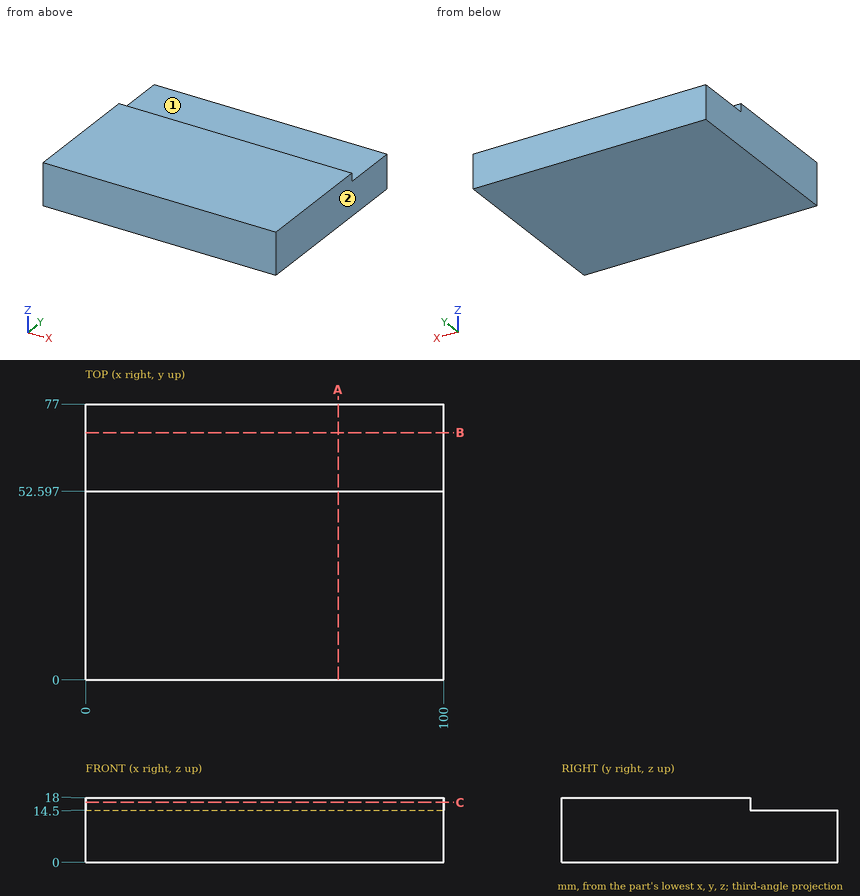
Study the drawing (mm; zero at the part's minimum x, y, z) and answer. A direction names the side the tool comes from. Give positions to 0.01 mm unless a question says otherwise; leave off trailing zeros. Order: outer loops, then holes, each group sorted by start corner. A loop starts at its lowest first (then second) coordinate and runs counter-clockwise, first axis right, second up. Notation, with made-up numbers: (49.25, 14) - (90.25, 14) arc R22 cw to (90.25, 40) - close; hole circle Ø9 at (-28.75, -37.75). An arc over 180 degrees is marked (long way). Use one line per item in the form item = value. Start each with the question number.
(1) A cutting plane is placed at A-A, the plane x = 70.5. Write down the section's boundary in (y, z).
(2) Consider line 1 (Z direction, x = 24, y = 66.5); line 2 (Y direction, x = 17, z = 17). Determine where each line is inside the solid, lowest interval first. Write a range as from..to.
(3) A cutting plane is placed at C-C, the plane z = 16.75. Write down the section's boundary in (x, y), then the cut area to 3 significant figures.
(4) A cutting plane is placed at B-B, the plane y = 69. Write down the section's boundary in (x, z).
(5) Flat-ended cylindrical pins translate along their axes: pin 1 Ø4 at (y, z) = (11.5, 4.5) entering from -X; pin 2 Ø1 at (x, z) = (49, 16) entering from +Y; pin 3 Ø7.5 at (x, y) = (29.5, 60.5) entering from +Z. Find the tip coordinate at first contact, or state that the pin passes through.
(6) For the marked faces 1 and 2, determine the directions among +Z, -Z, +X, -X, +Y, -Y from which every point of the face is accessible in a straight line to the end or side of a thin tool.
Ans:
q1.outline = (0, 0) - (77, 0) - (77, 14.5) - (52.6, 14.5) - (52.6, 18) - (0, 18) - close
q2.line_1 = 0..14.5
q2.line_2 = 0..52.6
q3.outline = (0, 0) - (100, 0) - (100, 52.6) - (0, 52.6) - close
q3.area = 5,260 mm^2
q4.outline = (0, 0) - (100, 0) - (100, 14.5) - (0, 14.5) - close
q5.pin_1 = 0
q5.pin_2 = 52.6
q5.pin_3 = 14.5
q6.face_1 = +Z, +X, -X, +Y
q6.face_2 = +Z, -Z, +X, +Y, -Y
